For this review, take the finished solid that the model builds, in its own axes (mm). A direction names the side the tool comes from. Give positions to 0.01 mm unless a question says otherwise; leave off trailing zeros. Write each loop counter-clockwise with the first axis right and the second up, starting at its lowest first coordinate (ties: lowest second). Pieces come first, ordered by that corner, then holes. Notation, with made-up numbers: M -9.5,6 L -4.5,6 A31 cw -4.5,36 Z; hole C 64,86.5 d10. An arc over 180 degrees is marked long. One line per item, written item: value. Start each with the question number.
Item 1: Consider section A-A, the plane z = 0. Write out the cut boundary in (x, y).
Item 2: Consider section D-D, the plane y = 71. Write out the cut boundary in (x, z), and give its area (3 significant figures).
Item 3: Clearance check with flat-ended pins moving along their axes: pin 1 Ø2 at (y, z) = (0.5, 66.5) entering from +X; pin 2 Ø4 at (x, z) = (-39, 112) entering from +Y; pin 3 Ø10 at (x, y) = (90, 228) entering from -Z; pin 4 Ø1.5 at (x, z) = (-41, -46) entering from -Y. State where each tip first meets the part, or that it passes through.
Item 4: Consider section C-C, the plane y = 138. Write out the cut boundary in (x, z), and give its area (3 significant figures).
Item 5: Mouldability with a two-part tool opening along X and no side actions: class faces 1 (the face through (-39.05, 1.01, -8.67)), 2 (the face through (-21.92, 116.57, 98.7)), 3 (the face through (25.99, 1.01, -77.15)), 4 (the face through (19, 0, -37)) as released by +X, released by -X, zero draft, split by the parting line, or undercut.
Item 6: To check wall thickness, follow probe 1 along X at (y, z) = (0.4, -70); probe 2 along Z at (x, y) = (-17, 287); probe 3 along X at (y, z) = (135.5, -62.5). State the ranges of each line that lie inside material, in increasing order.
Item 7: Consider section B-B, the plane x = 0. Write out the cut boundary in (y, z), and give its area (3 significant figures).
Item 8: Tool access review of faces 5 (the face through (-26.15, 1.01, 76.99)), 6 (the face through (-26.15, 1.01, -76.99)), 7 (the face through (38, 2, -19)), 8 (the face through (25.99, 1.01, 77.15)): name each direction out of +Z, -Z, +X, -X, +Y, -Y from which nothing blocks a thin tool from reaching the whole face with its end or side.
```python
from build123d import *

# Parameters (mm, degrees)
SKETCH1_W           = 88
SKETCH1_H           = 120
BOSS_EXTRUDE1_DEPTH = 2
SKETCH2_R           = 40
CUT_EXTRUDE1_DEPTH  = 2
SKETCH4_W           = 58
SKETCH4_H           = 20
SKETCH4_R           = 4.5
BOSS_EXTRUDE2_DEPTH = 2
FILLET1_R           = 10
FILLET2_R           = 2


# Read off the part's stored shape, not the designer's step: Thicken1
with BuildPart() as part:
    # Sketch1 → Boss-Extrude1 (new body)
    with BuildSketch(Plane(origin=(0, 0, 0), x_dir=(1, 0, 0), z_dir=(0, 1, 0))):
        Rectangle(SKETCH1_W, SKETCH1_H)
    extrude(amount=BOSS_EXTRUDE1_DEPTH)

    # Sketch2 → Cut-Extrude1 (cut)
    with BuildSketch(Plane(origin=(0, 2, 0), x_dir=(1, 0, 0), z_dir=(0, 1, 0))):
        with Locations(Location((0, 0, 0), (0, 0, 270))):
            Circle(SKETCH2_R)
    extrude(amount=-CUT_EXTRUDE1_DEPTH, mode=Mode.SUBTRACT)

    # Thicken1 outline → Thicken1 (revolve)
    with BuildSketch(Plane.XY):
        Polygon((201.764705882, 301.058823529), (200, 302), (40, 2), (42.266666667, 2), align=None)
    revolve(axis=Axis((0, 0, 0), (0, 1, 0)))

    # Sketch4 → Boss-Extrude2 (add)
    # profile 1 of 2: a face of its own
    with BuildSketch(Plane.XZ):
        with Locations((0, 70)):
            Rectangle(SKETCH4_W, SKETCH4_H)
        with Locations(Location((19, 70, 0), (0, 0, 270))):
            Circle(SKETCH4_R, mode=Mode.SUBTRACT)
        with Locations(Location((-19, 70, 0), (0, 0, 90))):
            Circle(SKETCH4_R, mode=Mode.SUBTRACT)
    # profile 2 of 2: a face of its own
    with BuildSketch(Plane.XZ):
        with Locations((0, -70)):
            Rectangle(SKETCH4_W, SKETCH4_H)
        with Locations(Location((-19, -70, 0), (0, 0, 270))):
            Circle(SKETCH4_R, mode=Mode.SUBTRACT)
        with Locations(Location((19, -70, 0), (0, 0, 90))):
            Circle(SKETCH4_R, mode=Mode.SUBTRACT)
    extrude(amount=-BOSS_EXTRUDE2_DEPTH)

    # Fillet1
    fillet1_edges = [part.edges().sort_by_distance(p)[0] for p in [
        (-29, 1, 80),
        (29, 1, 80),
        (29, 1, -80),
        (-29, 1, -80),
    ]]
    fillet(fillet1_edges, radius=FILLET1_R)

    # Fillet2
    fillet2_edges = [part.edges().sort_by_distance(p)[0] for p in [
        (44, 1, 60),
        (-44, 1, 60),
        (-44, 1, -60),
        (44, 1, -60),
    ]]
    fillet(fillet2_edges, radius=FILLET2_R)


solid = part.part
```
Model answer:
1. outline: M -201.76,301.06 L -42.27,2 L -44,2 L -44,0 L -40,0 L -40,2 L -200,302 Z; M 40,0 L 44,0 L 44,2 L 42.27,2 L 201.76,301.06 L 200,302 L 40,2 Z
2. outline: C 0,0 d158.13; hole C 0,0 d153.6
2. area: 1,110 mm2
3. pin 1: stops at x = 29
3. pin 2: stops at y = 153.12
3. pin 3: stops at z = -140.16
3. pin 4: stops at y = 0
4. outline: C 0,0 d229.6; hole C 0,0 d225.07
4. area: 1,620 mm2
5. face 1: undercut
5. face 2: undercut
5. face 3: released by +X
5. face 4: zero draft
6. probe 1: x = -29 to -23.5, -14.5 to 14.5, 23.5 to 29
6. probe 2: z = -193.52 to -191.25, 191.25 to 193.52
6. probe 3: x = -94.7 to -91.97, 91.97 to 94.7
7. outline: M 0,-80 L 2,-80 L 2,-42.27 L 301.06,-201.76 L 302,-200 L 2,-40 L 0,-40 Z; M 0,40 L 2,40 L 302,200 L 301.06,201.76 L 2,42.27 L 2,80 L 0,80 Z
7. area: 1,520 mm2
8. face 5: +Z, -X, -Y
8. face 6: -Z, -X, -Y
8. face 7: none
8. face 8: +Z, +X, -Y
